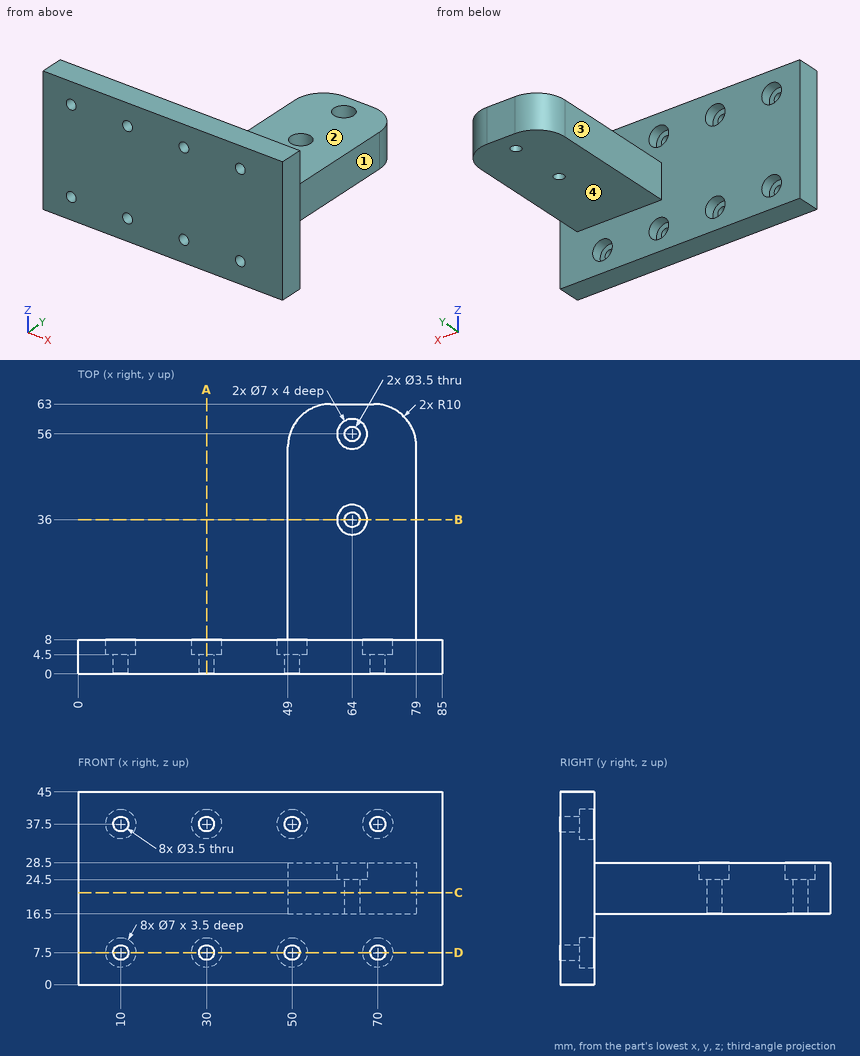
Verification items for this drawing (mm, ordinates from the low corner). A direction names the side the tool comes from. Coordinates: 2 decimals unless noted, no trailing zeros. Loops run counter-clockwise (first coordinate to the right, second up) from the corner with the lowest first, then second, coordinate; pieces in that order, holes last. Notation, with made-up numbers: (17.5, -13) - (73.5, -13) arc R10 ccw to (73.5, -4) - close; hole circle Ø3 at (-17, 23). An arc over 180 degrees is marked (long way). One line per item, written item: value. Start each with the question number.
(1) Cross-section at C-C on z = 21.5. Enter the section's corners in (x, y), plus the area to 3 significant figures.
(2) Depth check by flat-ended pin: P1, Ø3, axis at x = 70, z = 7.5, coming from the -Y side; P2, Ø1.5, axis at y = 51, z = 24.5, coming from the -X side; P3, Ø11, axis at x = 30, z = 37.5, coming from the +Y side; P4, Ø9, axis at x = 70, y = 48, coming from the -Z side. Enter the tip coordinate at first touch or a pass-through.
(3) Cross-section at B-B on y = 36. Enter the section's corners in (x, z).
(4) Tool access check on the marked faces 1, 2, 3 and 4. Record the directions out of +Z, -Z, +X, -X, +Y, -Y that give a thin tool (end or side, any length) a straight path to the whole face; none if there is none.
(5) Material ranges on line 1 (X direction, y = 7.15, z = 37.5); line 2 (X direction, y = 2.9, z = 37.5); line 3 (Y direction, x = 11, z = 3), recorded low to high. Write a range as [from, to].
(6) Cross-section at A-A on x = 30. Enter the section's corners in (y, z).
(7) Cross-section at D-D on z = 7.5. Count the separate pieces of the cut face and the enclosed holes in it, plus the area to 3 significant figures.
Results below:
1. outline: (0, 0) - (85, 0) - (85, 8) - (79, 8) - (79, 53) arc R10 ccw to (69, 63) - (59, 63) arc R10 ccw to (49, 53) - (49, 8) - (0, 8) - close; hole circle Ø3.5 at (64, 36); hole circle Ø3.5 at (64, 56)
1. area: 2,270 mm2
2. P1: passes through
2. P2: stops at x = 49
2. P3: stops at y = 8
2. P4: stops at z = 16.5
3. outline: (49, 16.5) - (62.25, 16.5) - (62.25, 24.5) - (60.5, 24.5) - (60.5, 28.5) - (49, 28.5) - close; (65.75, 16.5) - (79, 16.5) - (79, 28.5) - (67.5, 28.5) - (67.5, 24.5) - (65.75, 24.5) - close
4. face 1: +Z, -Z, +X, +Y
4. face 2: +Z, +X, -X, +Y
4. face 3: +Z, -Z, -X, +Y
4. face 4: -Z, +X, -X, +Y
5. line 1: x = [0, 6.5], [13.5, 26.5], [33.5, 46.5], [53.5, 66.5], [73.5, 85]
5. line 2: x = [0, 8.25], [11.75, 28.25], [31.75, 48.25], [51.75, 68.25], [71.75, 85]
5. line 3: y = [0, 8]
6. outline: (0, 0) - (8, 0) - (8, 4) - (4.5, 4) - (4.5, 5.75) - (0, 5.75) - close; (0, 9.25) - (4.5, 9.25) - (4.5, 11) - (8, 11) - (8, 34) - (4.5, 34) - (4.5, 35.75) - (0, 35.75) - close; (0, 39.25) - (4.5, 39.25) - (4.5, 41) - (8, 41) - (8, 45) - (0, 45) - close
7. separate pieces: 5
7. enclosed holes: 0
7. area: 519 mm2
